Source: CAD feature listing. Evaluate the final solid. Frame: model axes, mm. A direction names the side the tool comes from. Round coordinates to 2 decimals unless told otherwise and drop trailing zeros. Loops run counter-clockwise (first coordinate to the right, second up) from the corner with the lowest first, then second, coordinate; pieces in that order, holes last. Notation, with made-up numbers: M -21,86 L 11,86 A28 ccw 11,117 Z; hole C -1.75,76.25 d8. An arc over 180 degrees is marked long. One line per item, written item: value.
from build123d import *

# Parameters (mm, degrees)
FILLET4_R     = 0.5
CHAMFER1_SIZE = 1
FILLET6_R     = 0.75


with BuildPart() as part:
    # Sketch1 → Revolve1 (revolve)
    with BuildSketch(Plane.XY, mode=Mode.PRIVATE) as revolve1_sk:
        Polygon((0, 0), (1.75, 0), (1.75, 1.5), (1.25, 1.5), (1.25, 4.5), (9, 4.5), (9, 8.5), (2.5, 8.5), (2.5, 17.5), (0, 17.5), align=None)
    revolve(revolve1_sk.sketch.rotate(Axis((0, 8.13, 0), (0, -1, 0)), 90), axis=Axis((0, 8.13, 0), (0, -1, 0)))

    # Fillet4
    fillet4_edges = [part.edges().sort_by_distance(p)[0] for p in [
        (0, 8.5, -9),
        (0, 4.5, -9),
    ]]
    fillet(fillet4_edges, radius=FILLET4_R)

    # Chamfer1
    chamfer1_edges = [part.edges().sort_by_distance(p)[0] for p in [
        (0, 17.5, -2.5),
    ]]
    chamfer(chamfer1_edges, length=CHAMFER1_SIZE)

    # Fillet6
    # the kernel refuses this fillet: 0.75 mm, written as the material it takes off along each edge
    with BuildSketch(Plane(origin=(0, 1.5, 0), x_dir=(0, 0, 1), z_dir=(1, 0, 0))) as fillet6_piece_1:
        with BuildLine():
            CenterArc((1, 0.707106781), FILLET6_R, 289.471220634, 70.528779366)
            Line((1.75, 0.707106781), (1.765, 0.707106781))
            Line((1.765, 0.707106781), (1.765, 0))
            Line((1.765, 0), (1.75, -0.015))
            ThreePointArc((1.75, -0.015), (1.5, -0.015), (1.255, -0.014142136))
            Line((1.255, -0.014142136), (1.25, 0))
        make_face()
    revolve(axis=Axis((0, 1.5, 0), (0, -1, 0)), mode=Mode.SUBTRACT)
    with BuildSketch(Plane(origin=(0, 0, 0), x_dir=(0, 0, 1), z_dir=(1, 0, 0))) as fillet6_piece_2:
        with BuildLine():
            CenterArc((1.75 - FILLET6_R, -FILLET6_R), FILLET6_R, 0, 90)
            Line((1.75 - FILLET6_R, 0), (1.75 - FILLET6_R, FILLET6_R * 0.02))
            Line((1.75 - FILLET6_R, FILLET6_R * 0.02), (1.75 + FILLET6_R * 0.02, FILLET6_R * 0.02))
            Line((1.75 + FILLET6_R * 0.02, FILLET6_R * 0.02), (1.75 + FILLET6_R * 0.02, -FILLET6_R))
            Line((1.75 + FILLET6_R * 0.02, -FILLET6_R), (1.75, -FILLET6_R))
        make_face()
    revolve(axis=Axis((0, 0, 0), (0, -1, 0)), mode=Mode.SUBTRACT)


solid = part.part
1. Reachability of faces 4 (the face through (2, 8.5, 2)), 5 (the face through (0, 0, 0)) from +Z, -Z, +X, -X, +Y, -Y: full face, straight path, thin tool, end or side. Return the list, or none.
Report:
face 4: +Y
face 5: +Z, -Z, +X, -X, -Y
2. Ray query, line 1 (Y direction, x = 5.25, z = 0); line 2 (X direction, y = 5, z = 0.25); line 3 (Z direction, x = -2, y = 14.25). Return the intervals inside material, ascending. Write a range as [from, to].
Report:
line 1: y = [4.5, 8.5]
line 2: x = [-9, 9]
line 3: z = [-1.5, 1.5]
3. Section query A-A (x = 0). Return the cut outline in (y, z), and give its area (3 significant figures).
Report:
outline: M 0,-1 A0.75 ccw 0.75,-1.75 L 0.79,-1.75 A0.75 ccw 1.5,-1.25 L 4.5,-1.25 L 4.5,-8.5 A0.5 ccw 5,-9 L 8,-9 A0.5 ccw 8.5,-8.5 L 8.5,-2.5 L 16.5,-2.5 L 17.5,-1.5 L 17.5,1.5 L 16.5,2.5 L 8.5,2.5 L 8.5,8.5 A0.5 ccw 8,9 L 5,9 A0.5 ccw 4.5,8.5 L 4.5,1.25 L 1.5,1.25 A0.75 ccw 0.79,1.75 L 0.75,1.75 A0.75 ccw 0,1 Z
area: 128 mm2
4. Pin query (flat end, axial travel): pin 1 (2 mm diameter, centred on x = 1.5, y = 11.5, fed in from -Z); pin 2 (1.5 mm diameter, centred on y = 7.5, z = 1, fed in from -X); pin 3 (1 mm diameter, centred on x = 3, z = -2, fed in from +Y). Return the tip coordinate at first contact, or that it passes through.
Report:
pin 1: stops at z = -2.45
pin 2: stops at x = -9
pin 3: stops at y = 8.5
5. Pull-direction query (Y, two-part tool) for faces 1 (the face through (-0.1, 12.6, -2.5)), 2 (the face through (-2, 17, 0)), 3 (the face through (-0.05, 3.02, -1.25)); classes: released by +Y, released by -Y, zero draft, split by the parting line, or undercut.
Report:
face 1: zero draft
face 2: released by +Y
face 3: undercut
6. Section query D-D (y = 13.75). Return the cut outline in (x, z), and give its area (3 significant figures).
Report:
outline: C 0,0 d5
area: 19.6 mm2
7. Section query C-C (y = 5.75). Return the cut outline in (x, z), and give its area (3 significant figures).
Report:
outline: C 0,0 d18
area: 254 mm2
8. Section query B-B (z = 0). Return the cut outline in (x, y).
Report:
outline: M -9,5 A0.5 ccw -8.5,4.5 L -1.25,4.5 L -1.25,1.5 A0.75 ccw -1.75,0.79 L -1.75,0.75 A0.75 ccw -1,0 L 1,0 A0.75 ccw 1.75,0.75 L 1.75,0.79 A0.75 ccw 1.25,1.5 L 1.25,4.5 L 8.5,4.5 A0.5 ccw 9,5 L 9,8 A0.5 ccw 8.5,8.5 L 2.5,8.5 L 2.5,16.5 L 1.5,17.5 L -1.5,17.5 L -2.5,16.5 L -2.5,8.5 L -8.5,8.5 A0.5 ccw -9,8 Z
